```python
from build123d import *

# Parameters (mm, degrees)
SKETCH283_R     = 2.5
SKETCH283_R_2   = 0.5
PAD192_DEPTH    = 1
SKETCH277_R     = 0.97
SKETCH277_R_2   = 0.55
PAD187_DEPTH    = 1.5
SKETCH309_R     = 2.5
SKETCH309_R_2   = 1.5
PAD214_DEPTH    = 4
CHAMFER006_SIZE = 0.95


with BuildPart() as part:
    # Sketch283 → Pad192 (new body)
    with BuildSketch(Plane.XY):
        Circle(SKETCH283_R)
        Circle(SKETCH283_R_2, mode=Mode.SUBTRACT)
    extrude(amount=PAD192_DEPTH)

    # Sketch277 (on Face4 of Pad192) → Pad187 (join)
    with BuildSketch(Plane.XY.offset(1)):
        Circle(SKETCH277_R)
        Circle(SKETCH277_R_2, mode=Mode.SUBTRACT)
    extrude(amount=PAD187_DEPTH)

    # Sketch309 (on Face2 of Pad187) → Pad214 (join)
    with BuildSketch(Plane(origin=(0, 0, 0), x_dir=(1, 0, 0), z_dir=(0, 0, -1))):
        Circle(SKETCH309_R)
        Circle(SKETCH309_R_2, mode=Mode.SUBTRACT)
    extrude(amount=PAD214_DEPTH)

    # Chamfer006
    chamfer006_edges = [part.edges().sort_by_distance(p)[0] for p in [
        (-1.5, 0, 0),
    ]]
    chamfer(chamfer006_edges, length=CHAMFER006_SIZE)


with BuildPart() as part_1:
    # Body056 placement: moved
    add(part.part.moved(Location((0, 0, -2.2))))


solid = part_1.part
```
Design review of the part built by this model. Coordinates are the model's own, in mm. A direction names the side the tool comes from. Coordinates: 2 decimals unless noted, no trailing zeros. Write each loop counter-clockwise with the first axis right and the second up, starting at its lowest first coordinate (ties: lowest second). Pieces come first, ordered by that corner, then holes.
1) Mouldability with a two-part tool opening along Y and no side actions: class faces 4 (the cylindrical face through (-0.108, -0.488, -1.707)), 5 (the cylindrical face through (-0.21, -0.947, -0.461)), 6 (the flat face through (1, -1, -1.2)) as +Y half, -Y half, draft (parallel to the pull), parting line (faces both ways), or undercut.
2) Insertion check: pin 1 (2 mm diameter, centred on x = -1, y = -0.5, fed in from -Z); pin 2 (1.8 mm diameter, centred on x = 0, y = 0, fed in from -Z). Each pin has a flat end and moves straight along its axis. Give the tip position at first contact, or say it passes through.
3) Add section A-A (y = 0). Write out the cut boundary in (x, z).
4) Add section D-D (y = -2.15). Write out the cut boundary in (x, z).
5) Add section C-C (z = -2.5). Write out the cut boundary in (x, y).
6) Machinability: for faces 1 (the cylindrical face through (-0.54, 2.44, -3.66)), 2 (the cylindrical face through (0.525, 0.165, -0.461)), 3 (the cylindrical face through (-1.5, -0.07, -4.65)), which of the approach directions +Z, -Z, +X, -X, +Y, -Y give a long, thin tool a straight path to every point of the face, cutting with its end or side? Answer none if there is none.
7) To check wall thickness, follow L1, parallel to X at y = 0, z = -4.65; L2, parallel to X at y = 0.05, z = -1.5; L3, parallel to Y at x = 0.85, z = -4. State the ranges of each line that lie inside material, in increasing order.
Check result:
1. face 4: undercut
1. face 5: parting line
1. face 6: draft
2. pin 1: stops at z = -6.2
2. pin 2: stops at z = -2.55
3. outline: (-2.5, -6.2) - (-1.5, -6.2) - (-1.5, -3.15) - (-0.55, -2.2) - (-0.5, -2.2) - (-0.5, -1.2) - (-0.55, -1.2) - (-0.55, 0.3) - (-0.97, 0.3) - (-0.97, -1.2) - (-2.5, -1.2) - close; (0.5, -2.2) - (0.55, -2.2) - (1.5, -3.15) - (1.5, -6.2) - (2.5, -6.2) - (2.5, -1.2) - (0.97, -1.2) - (0.97, 0.3) - (0.55, 0.3) - (0.55, -1.2) - (0.5, -1.2) - close
4. outline: (-1.28, -6.2) - (1.28, -6.2) - (1.28, -1.2) - (-1.28, -1.2) - close
5. outline: circle Ø5 at (0, 0); hole circle Ø1.7 at (0, 0)
6. face 1: +Z, -Z
6. face 2: +Z
6. face 3: -Z
7. L1: x = -2.5 to -1.5, 1.5 to 2.5
7. L2: x = -2.5 to -0.5, 0.5 to 2.5
7. L3: y = -2.35 to -1.24, 1.24 to 2.35
